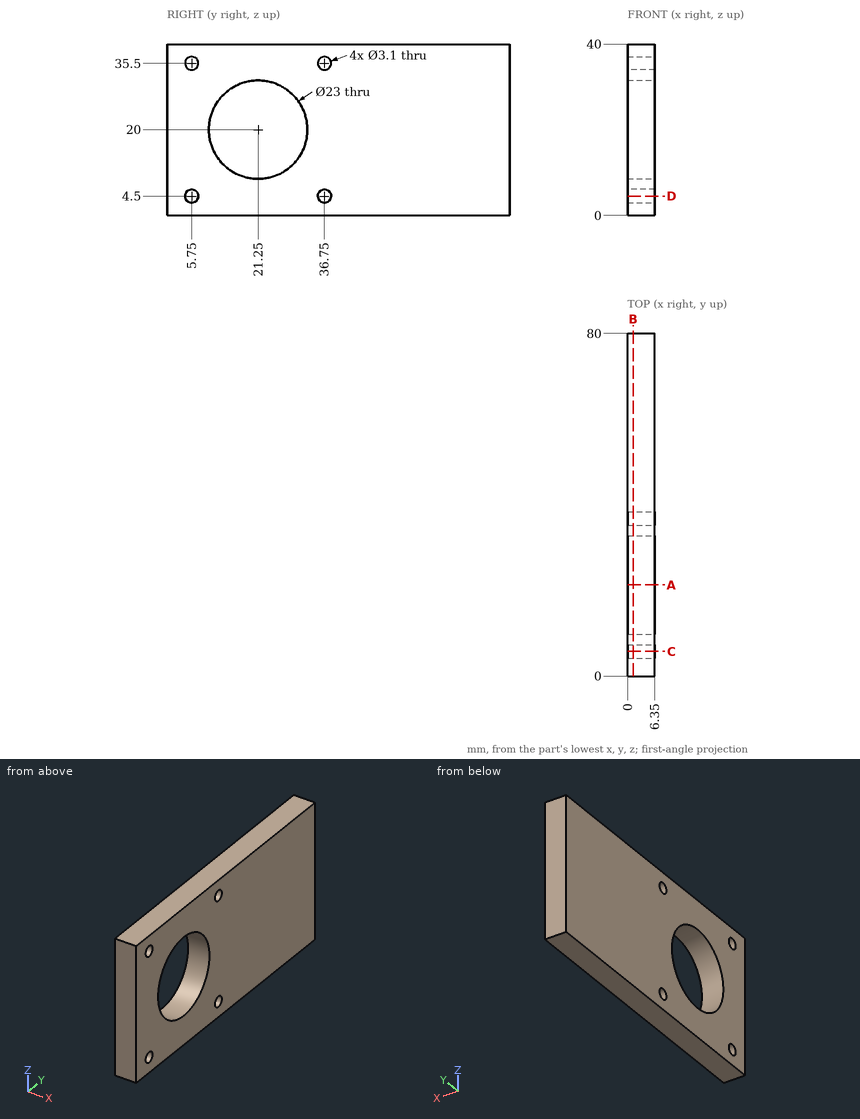
Could you check a few things on this drawing? It's one solid part, dimensions in mm from its lowest x, y, z. Give positions to 0.01 mm unless a question says otherwise; leave off trailing zeros. Loops run counter-clockwise (first coordinate to the right, second up) from the corner with the lowest first, then second, coordinate; pieces in that order, holes last. Notation, with made-up numbers: M -39,-36 L -32,-36 A19 ccw -32,-5 Z; hole C 43,65 d1. An arc over 180 degrees is marked long. Answer as a JSON object with one key per item and string values.
Q1. Suppose I cut it at A-A, the plane y = 21.25. List the corners of the cut face in (x, z) for me.
Values found:
{"outline": "M 0,0 L 6.35,0 L 6.35,8.5 L 0,8.5 Z; M 0,31.5 L 6.35,31.5 L 6.35,40 L 0,40 Z"}
Q2. For P1, Ø2, axis at y = 33, z = 14, coming from the -X side; P2, Ø3, axis at y = 5.75, z = 35.5, coming from the -X side, each with a flat end and sliding along its axis, tell me the tip position at first contact or that it passes through.
Values found:
{"P1": "stops at x = 0", "P2": "passes through"}
Q3. Suppose I cut it at D-D, the plane z = 4.5. List the corners of the cut face in (x, y) for me.
Values found:
{"outline": "M 0,0 L 6.35,0 L 6.35,4.2 L 0,4.2 Z; M 0,7.3 L 6.35,7.3 L 6.35,35.2 L 0,35.2 Z; M 0,38.3 L 6.35,38.3 L 6.35,80 L 0,80 Z"}
Q4. Suppose I cut it at B-B, the plane x = 1.25. List the corners of the cut face in (y, z) for me, plus the area to 3 significant figures.
Values found:
{"outline": "M 0,0 L 80,0 L 80,40 L 0,40 Z; hole C 5.75,4.5 d3.1; hole C 5.75,35.5 d3.1; hole C 21.25,20 d23; hole C 36.75,4.5 d3.1; hole C 36.75,35.5 d3.1", "area": "2,750 mm²"}
Q5. If I drill on probe 1 along Y at (x, z) = (4, 4.5); probe 2 along Y at (x, z) = (2.75, 19.5); probe 3 along Y at (x, z) = (3, 4), over which ranges is the centre line in solid material (lowest first)? Write a range as [from, to].
Values found:
{"probe 1": "y = [0, 4.2], [7.3, 35.2], [38.3, 80]", "probe 2": "y = [0, 9.76], [32.74, 80]", "probe 3": "y = [0, 4.28], [7.22, 35.28], [38.22, 80]"}
Q6. Suppose I cut it at C-C, the plane y = 5.75. List the corners of the cut face in (x, z) for me, plus the area to 3 significant figures.
Values found:
{"outline": "M 0,0 L 6.35,0 L 6.35,2.95 L 0,2.95 Z; M 0,6.05 L 6.35,6.05 L 6.35,33.95 L 0,33.95 Z; M 0,37.05 L 6.35,37.05 L 6.35,40 L 0,40 Z", "area": "215 mm²"}
